Input: part model. Units: mm. Frame: model coordinates. A direction names the side the tool comes from. Coordinates: 2 decimals unless noted, no trailing zeros. Write each loop counter-clockwise with the first axis right and the second up, starting at its lowest first coordinate (ties: lowest second). Pieces come first, ordered by that corner, then holes. Notation, with made-up numbers: (53, 53.5) - (109, 53.5) arc R24 cw to (109, 69.5) - close; hole circle Ø10 at (38.25, 26). An arc over 180 degrees is marked (long way). Put each result on its own line as item: value. Start each with the question number.
1. Cut plane A-A, the plane z = 9.82. Return loops of the section in (x, y), and give its area (3 significant figures).
2. Cut plane C-C, the plane x = 43.75. Return loops of the section in (y, z).
3. Cut plane D-D, the plane z = 3. Return loops of the section in (x, y), and give its area (3 significant figures).
4. Access query for faces 1 (the flat face through (36, -4.75, 33)), 2 (the flat face through (4, 15.25, 9)), 3 (the cylindrical face through (-50.39, -18.15, 19.72)). Directions: +Z, -Z, +X, -X, +Y, -Y. A direction counts if a zero-diameter tool reaches every point of the face in a straight line with its end or side. Return the directions, or none.
5. Cut plane B-B, the plane y = -19.5. Return loops of the section in (x, z).
6. Pull-direction query (Z, two-part tool) for faces 4 (the cylindrical face through (-54.9, -0.3, 12.3)), 5 (the flat face through (36, 4.75, 33)), 6 (the flat face through (38.1, 0.1, 25)); classes: released by +Z, released by -Z, zero draft, split by the parting line, or undercut.
7. Pin query (flat end, axial travel): pin 1 (5 mm diameter, centred on x = 36.25, y = 0, fed in from +Z); pin 2 (5.5 mm diameter, centred on y = 0, z = 11, fed in from +X); pin 3 (4 mm diameter, centred on x = 42, y = -5, fed in from -Z). Return the tip coordinate at first contact, or that it passes through.
8. Line query: line 1 (X direction, y = 19.5, z = 29); line 2 (Y direction, x = -51.25, z = 22.5); line 3 (X direction, y = 2, z = 37.5). Output: solid intervals per line, ascending.
from build123d import *

# Parameters (mm, degrees)
SKETCH_W        = 117.5
SKETCH_H        = 50
PAD_DEPTH       = 40
POCKET_DEPTH    = 18
SKETCH002_R     = 1.6
POCKET001_DEPTH = 40.001
SKETCH003_W     = 17.5
SKETCH003_H     = 9.5
POCKET002_DEPTH = 15
SKETCH004_R     = 1.6
POCKET003_DEPTH = 25.001
SKETCH006_R     = 2.5
POCKET004_DEPTH = 117.501


with BuildPart() as part:
    # Sketch → Pad (new body)
    with BuildSketch(Plane.XY):
        Rectangle(SKETCH_W, SKETCH_H)
    extrude(amount=PAD_DEPTH)

    # Sketch001 → Pocket (cut, symmetric)
    with BuildSketch(Plane.XY):
        Polygon((56.75, -13), (58.75, -13), (58.75, 13), (56.75, 13), (56.75, 15.25), (-51.25, 15.25), (-51.25, -15.25), (56.75, -15.25), align=None)
    extrude(amount=POCKET_DEPTH, both=True, mode=Mode.SUBTRACT)

    # Sketch002 → Pocket001 (cut, through all)
    with BuildSketch(Plane.XY):
        with Locations((-51.25, 19.5)):
            Circle(SKETCH002_R)
        with Locations((43.75, 19.5)):
            Circle(SKETCH002_R)
        with Locations((-51.25, -19.5)):
            Circle(SKETCH002_R)
        with Locations((43.75, -19.5)):
            Circle(SKETCH002_R)
    extrude(amount=POCKET001_DEPTH, mode=Mode.SUBTRACT)

    # Sketch003 (on Face5 of Pocket001) → Pocket002 (cut)
    with BuildSketch(Plane.XY.offset(40)):
        with Locations((36.25, 0)):
            Rectangle(SKETCH003_W, SKETCH003_H)
    extrude(amount=-POCKET002_DEPTH, mode=Mode.SUBTRACT)

    # Sketch004 (on Face23 of Pocket002) → Pocket003 (cut, through all)
    with BuildSketch(Plane.XY.offset(25)):
        with Locations((36.25, 0)):
            Circle(SKETCH004_R)
    extrude(amount=-POCKET003_DEPTH, mode=Mode.SUBTRACT)

    # Sketch006 (on DatumPlane) → Pocket004 (cut, through all)
    with BuildSketch(Plane.YZ.offset(58.75)):
        with Locations((0, 9.82)):
            Circle(SKETCH006_R)
    extrude(amount=-POCKET004_DEPTH, mode=Mode.SUBTRACT)


solid = part.part
Report:
1. outline: (-58.75, -25) - (58.75, -25) - (58.75, -13) - (56.75, -13) - (56.75, -15.25) - (-51.25, -15.25) - (-51.25, -2.5) - (-58.75, -2.5) - close; (-58.75, 2.5) - (-51.25, 2.5) - (-51.25, 15.25) - (56.75, 15.25) - (56.75, 13) - (58.75, 13) - (58.75, 25) - (-58.75, 25) - close; hole circle Ø3.2 at (-51.25, -19.5); hole circle Ø3.2 at (-51.25, 19.5); hole circle Ø3.2 at (43.75, -19.5); hole circle Ø3.2 at (43.75, 19.5)
1. area: 2,460 mm^2
2. outline: (-25, 0) - (-21.1, 0) - (-21.1, 40) - (-25, 40) - close; (-17.9, 0) - (-15.25, 0) - (-15.25, 18) - (15.25, 18) - (15.25, 0) - (17.9, 0) - (17.9, 40) - (4.75, 40) - (4.75, 25) - (-4.75, 25) - (-4.75, 40) - (-17.9, 40) - close; (21.1, 0) - (25, 0) - (25, 40) - (21.1, 40) - close
3. outline: (-58.75, -25) - (58.75, -25) - (58.75, -13) - (56.75, -13) - (56.75, -15.25) - (-51.25, -15.25) - (-51.25, 15.25) - (56.75, 15.25) - (56.75, 13) - (58.75, 13) - (58.75, 25) - (-58.75, 25) - close; hole circle Ø3.2 at (-51.25, -19.5); hole circle Ø3.2 at (-51.25, 19.5); hole circle Ø3.2 at (43.75, -19.5); hole circle Ø3.2 at (43.75, 19.5)
3. area: 2,500 mm^2
4. face 1: +Z
4. face 2: -Z
4. face 3: +Z, -Z
5. outline: (-58.75, 0) - (-52.85, 0) - (-52.85, 40) - (-58.75, 40) - close; (-49.65, 0) - (42.15, 0) - (42.15, 40) - (-49.65, 40) - close; (45.35, 0) - (58.75, 0) - (58.75, 40) - (45.35, 40) - close
6. face 4: undercut
6. face 5: zero draft
6. face 6: released by +Z
7. pin 1: stops at z = 25
7. pin 2: stops at x = -51.25
7. pin 3: stops at z = 18
8. line 1: x = -58.75 to -52.85, -49.65 to 42.15, 45.35 to 58.75
8. line 2: y = -25 to -21.1, -17.9 to 17.9, 21.1 to 25
8. line 3: x = -58.75 to 27.5, 45 to 58.75
